Work out the finished part from the listing and answer in its coordinate system (mm). Give positions to 0.01 mm unless a question says otherwise; leave off trailing zeros. Loops run counter-clockwise (first coordinate to the right, second up) from the corner with the lowest first, then second, coordinate; pieces in that order, holes last. Notation, with made-up numbers: (-8.5, -10) - (45.5, -10) arc R21 ccw to (45.5, 0) - close; hole circle Ø7 at (76, -37.5). An arc over 180 degrees is marked (long way). One line per question, with ' | ' between items. Start each with the question number.
1. Section B-B (z = -4.5) is taken. Determine the outline of the cut face in (x, y), plus the area to 3 significant figures.
2. Section C-C (x = -4.5) is taken. Determine the outline of the cut face in (y, z), plus the area to 3 significant figures.
3. Section A-A (y = 2) is taken. Determine the outline of the cut face in (x, z).
4. Find the intervals of material crossed by line 1 (Y direction, x = 0, z = -4.25); line 2 (Z direction, x = 0, y = 3); line 3 (Y direction, x = 1, z = -5.75), in increasing order.
5. Each of these flat-tipped pins is pushed along its axis until it touches: pin 1 (6 mm diameter, centred on x = 0.5, y = 29.5, fed in from -Z); pin 2 (1.5 mm diameter, centred on x = -1, z = 4.5, fed in from +Y). Where does it stop, or does it pass through?
6. For a pull along X with two mould halves and no side action, classify faces 1 (the face through (2.435, 6.761, -0.767)), 2 (the face through (0.096, 14.602, 0.433)), 3 (the face through (0.1, 38.1, 0.1)), 4 (the face through (-6.35, 16, 0)) as released by +X, released by -X, zero draft, split by the parting line, or undercut.
from build123d import *

# Parameters (mm, degrees)
BOSS_EXTRUDE1_DEPTH         = 9.398
F_1_4_0_249_DOWEL_HOLE1_D   = 6.3246
F_1_4_20_TAPPED_HOLE1_D     = 5.1054
F_1_4_20_TAPPED_HOLE1_DEPTH = 13.335
F_1_4_20_TAPPED_HOLE1_TIP   = 1.533816902


with BuildPart() as part:
    # Sketch2 → Boss-Extrude1 (new body, symmetric)
    with BuildSketch(Plane.XY):
        with BuildLine():
            Line((-6.35, 0), (6.35, 0))
            Line((6.35, 0), (6.35, 31.75))
            ThreePointArc((6.35, 31.75), (0, 38.1), (-6.35, 31.75))
            Line((-6.35, 31.75), (-6.35, 0))
        make_face()
    extrude(amount=BOSS_EXTRUDE1_DEPTH, both=True)

    # 1/4 (0.249) Dowel Hole1 (through all)
    with Locations(Plane.XY.offset(9.398)):
        with Locations((0, 31.75)):
            Hole(F_1_4_0_249_DOWEL_HOLE1_D / 2)

    # 1/4-20 Tapped Hole1
    with Locations(Plane(origin=(0, 0, 0), x_dir=(-1, 0, 0), z_dir=(0, -1, 0))):
        with Locations((0, 0)):
            Hole(F_1_4_20_TAPPED_HOLE1_D / 2, depth=F_1_4_20_TAPPED_HOLE1_DEPTH)
            with Locations((0, 0, -(F_1_4_20_TAPPED_HOLE1_DEPTH + F_1_4_20_TAPPED_HOLE1_TIP / 2))):  # 118° drill point
                Cone(0, F_1_4_20_TAPPED_HOLE1_D / 2, F_1_4_20_TAPPED_HOLE1_TIP, mode=Mode.SUBTRACT)


solid = part.part
Conclusion:
1) outline: (-6.35, 0) - (6.35, 0) - (6.35, 31.75) arc R6.35 ccw to (-6.35, 31.75) - close; hole circle Ø6.32 at (0, 31.75) | area: 435 mm²
2) outline: (0, -9.4) - (36.23, -9.4) - (36.23, 9.4) - (0, 9.4) - close | area: 681 mm²
3) outline: (-6.35, -9.4) - (6.35, -9.4) - (6.35, 9.4) - (-6.35, 9.4) - close; hole circle Ø5.11 at (0, 0)
4) line 1: 0 to 28.59, 34.91 to 38.1 | line 2: -9.4 to -2.55, 2.55 to 9.4 | line 3: 0 to 28.75, 34.75 to 38.02
5) pin 1: z = -9.4 | pin 2: y = 38.1
6) face 1: undercut | face 2: undercut | face 3: split by the parting line | face 4: released by -X
